```python
from build123d import *

# Parameters (mm, degrees)
BOSS_EXTRUDE1_DEPTH = 177.8
SKETCH2_W           = 101.6
SKETCH2_H           = 838.2


with BuildPart() as part:
    # Sketch1 → Boss-Extrude1 (new body)
    with BuildSketch(Plane.XY.offset(1016)):
        Polygon((-102.652877862, -177.8), (102.652877862, -177.8), (205.305755724, 0), (102.652877862, 177.8), (-102.652877862, 177.8), (-205.305755724, 0), align=None)
    extrude(amount=-BOSS_EXTRUDE1_DEPTH)

    # Sketch2 → Revolve1 (revolve)
    with BuildSketch(Plane(origin=(0, 0, 0), x_dir=(1, 0, 0), z_dir=(0, 1, 0))):
        with Locations((50.8, -419.1)):
            Rectangle(SKETCH2_W, SKETCH2_H)
    revolve(axis=Axis((0, 0, 0), (0, 0, 1)))


solid = part.part
```
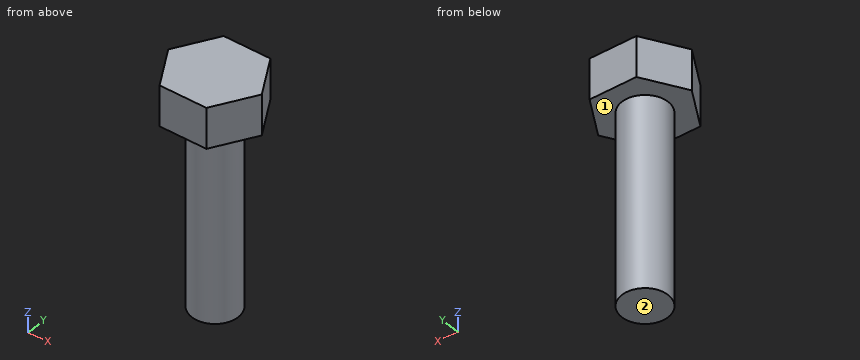
The listing builds one solid part. Answer for the finished solid, in the listing's coordinates (mm). Face numbers are marked on the shaded views. A direction names the side the tool comes from. Round coordinates to 2 decimals unless told otherwise and drop trailing zeros. Write each loop counter-clockwise with the first axis right and the second up, starting at its lowest first coordinate (ties: lowest second). Pieces come first, ordered by that corner, then holes. Notation, with made-up numbers: (11, -37.75) -> (44, -37.75) arc R24 cw to (44, -21.75) -> close; hole circle Ø3 at (38, 26.25). An arc over 180 degrees is marked (long way). Answer as a JSON object with one key per item and string values. Group by question number.
Q1. Section A-A (x = 0) is taken. Write down the section's boundary in (y, z).
Q2. Which of the six approach directions +Z, -Z, +X, -X, +Y, -Y give full straight-line access (tool end or side, diameter ignored) to the marked faces 1 and 2?
Q3. Section B-B (z = 683) is taken. Write down the section's boundary in (x, y).
Q4. Straight lines are drawn through the part: line 1 along Z through (x, y) = (170.5, 13.5); line 2 along Y through (x, z) = (20, 61.5); line 3 along Y through (x, z) = (-87, 502). For each, find the intervals that lie inside material, in ascending order.
Q5. Each of these flat-tipped pins is pushed along its axis until it touches: pin 1 Ø1.5 at (y, z) = (-126, 899.5) entering from +X; pin 2 Ø5 at (x, y) = (131.5, -54.5) entering from -Z; pin 3 Ø2 at (x, z) = (10, 312.5) entering from -Y. Where does it stop, or does it pass through?
Q6. Section C-C (y = -53) is taken. Write down the section's boundary in (x, z).
Check values:
{
 "1": {"outline": "(-177.8, 838.2) -> (-101.6, 838.2) -> (-101.6, 0) -> (101.6, 0) -> (101.6, 838.2) -> (177.8, 838.2) -> (177.8, 1016) -> (-177.8, 1016) -> close"},
 "2": {"face 1": "-Z", "face 2": "-Z, +X, -X, +Y, -Y"},
 "3": {"outline": "circle Ø203.2 at (0, 0)"},
 "4": {"line 1": "838.2 to 1016", "line 2": "-99.61 to 99.61", "line 3": "-52.47 to 52.47"},
 "5": {"pin 1": "x = 132.99", "pin 2": "z = 838.2", "pin 3": "y = -101.2"},
 "6": {"outline": "(-174.71, 838.2) -> (-86.68, 838.2) -> (-86.68, 0) -> (86.68, 0) -> (86.68, 838.2) -> (174.71, 838.2) -> (174.71, 1016) -> (-174.71, 1016) -> close"}
}
